```python
from build123d import *

# Parameters (mm, degrees)
F0_W     = 19.05
F0_H     = 12.7
F1_DEPTH = 12.7
F2_T     = -1.27
F3_R     = 4.7625
F4_DEPTH = 1.27
F5_R     = 1.27
F6_DEPTH = 1.27


with BuildPart() as f1:
    # F0 (on Top) → F1 (new body)
    with BuildSketch(Plane.XY):
        Rectangle(F0_W, F0_H)
    extrude(amount=F1_DEPTH)

    # F2
    f2_openings = [f1.faces().sort_by_distance(p)[0] for p in [
        (0, 0, 12.7),
    ]]
    offset(amount=F2_T, openings=f2_openings)

    # F3 (on face) → F4 (cut, through all)
    with BuildSketch(Plane.YZ.offset(9.525)):
        with Locations((0, 6.35)):
            Circle(F3_R)
    extrude(amount=-F4_DEPTH, mode=Mode.SUBTRACT)

    # F5 (on face) → F6 (cut, through all)
    with BuildSketch(Plane(origin=(-9.525, 0, 0), x_dir=(0, -1, 0), z_dir=(-1, 0, 0))):
        with Locations((-2.38125, 6.35)):
            Circle(F5_R)
        with Locations((2.38125, 6.35)):
            Circle(F5_R)
    extrude(amount=-F6_DEPTH, mode=Mode.SUBTRACT)


solid = f1.part
```
Input: part model. Units: mm. Frame: model coordinates. A direction names the side the tool comes from. Coordinates: 2 decimals unless noted, no trailing zeros. Loops run counter-clockwise (first coordinate to the right, second up) from the corner with the lowest first, then second, coordinate; pieces in that order, holes last. Notation, with made-up numbers: (39.5, 51.25) -> (50.5, 51.25) arc R13 cw to (50.5, 59.25) -> close; hole circle Ø10 at (83, 34.25). An arc over 180 degrees is marked (long way). Use a Markdown table: item, result.
1) Cut plane C-C (x = -2). Return the cut outline in (y, z).
Results found:
| item | result |
|---|---|
| outline | (-6.35, 0) -> (6.35, 0) -> (6.35, 12.7) -> (5.08, 12.7) -> (5.08, 1.27) -> (-5.08, 1.27) -> (-5.08, 12.7) -> (-6.35, 12.7) -> close |
2) Access query for faces 1 (the cylindrical face through (8.9, -1.03, 1.7)), 2 (the cylindrical face through (-8.9, -2.22, 7.61)), 3 (the flat face through (0, -5.08, 7)). Directions: +Z, -Z, +X, -X, +Y, -Y. A direction counts if a zero-diameter tool reaches every point of the face in a straight line with its end or side. Return the directions, or none.
Results found:
| item | result |
|---|---|
| face 1 | +X |
| face 2 | +X, -X |
| face 3 | +Z |
3) Pull-direction query (Y, two-part tool) for faces 4 (the flat face through (8.255, -2, 11)), 5 (the flat face through (0, 0, 0)), 6 (the flat face through (0, 6.35, 6)); classes: released by +Y, released by -Y, zero draft, split by the parting line, or undercut.
Results found:
| item | result |
|---|---|
| face 4 | undercut |
| face 5 | zero draft |
| face 6 | released by +Y |
4) Cut plane B-B (z = 6.35). Give the number of separate pieces and of enclosed holes in the cut face, then the cut area to 3 significant figures.
Results found:
| item | result |
|---|---|
| separate pieces | 3 |
| enclosed holes | 0 |
| area | 55.6 mm2 |
5) Contact query for flat-ended pins moving along their axis: pin 1 (1.5 mm diameter, centred on y = -2.38, z = 6.35, fed in from +X); pin 2 (1.5 mm diameter, centred on y = -2.5, z = 7.5, fed in from +X) (3 decimals); pin 3 (3 mm diameter, centred on x = -4, y = -2.5, fed in from +Z). Output: stop coordinate, or through.
Results found:
| item | result |
|---|---|
| pin 1 | passes through |
| pin 2 | stops at x = -8.255 |
| pin 3 | stops at z = 1.27 |
6) Cut plane D-D (y = -2.25). Return the cut outline in (x, z) (3 decimals), then the cut area to 3 significant figures.
Results found:
| item | result |
|---|---|
| outline | (-9.525, 0) -> (9.525, 0) -> (9.525, 2.153) -> (8.255, 2.153) -> (8.255, 1.27) -> (-8.255, 1.27) -> (-8.255, 5.087) -> (-9.525, 5.087) -> close; (-9.525, 7.613) -> (-8.255, 7.613) -> (-8.255, 12.7) -> (-9.525, 12.7) -> close; (8.255, 10.547) -> (9.525, 10.547) -> (9.525, 12.7) -> (8.255, 12.7) -> close |
| area | 39.4 mm2 |
7) Material intervals for line 1 along Y through (x, z) = (-1.75, 11); line 2 along X through (y, z) = (-4, 9.25) (3 decimals); line 3 along Z through (x, y) = (4.5, 0.5), sorted ascending. Write a range as from..to.
Results found:
| item | result |
|---|---|
| line 1 | y = -6.35..-5.08, 5.08..6.35 |
| line 2 | x = -9.525..-8.255, 8.255..9.525 |
| line 3 | z = 0..1.27 |
